Drawing for the job (mm, zero at the part's lowest x, y, z). A direction names the side the tool comes from. Coordinates: 2 decimals unless noted, no trailing zeros. Order: outer loops, then holes, each group sorted by start corner. A loop starts at its lowest first (then second) coordinate and runs counter-clockwise, first axis right, second up.
1) Cut at D-D (x = 9.5). List the corners of the cut face in (y, z).
2) Pin check, flat tips, straight feed: pin 1 Ø2 at (x, z) = (110, 4.5) entering from +Y; pin 2 Ø3 at (x, z) = (20.5, 30.5) entering from -Y; pin 3 Ø1.5 at (x, y) = (98, 18.5) entering from -Z; pin 4 Ø2 at (x, z) = (91, 26) entering from +Y. Stop position of each tip, or through.
3) Wall check: L1, parallel to X at y = 17, z = 19; L2, parallel to Y at x = 111, z = 18.5; L3, parallel to Z at x = 9, y = 24. Give the ranges that are in metal, low to high.
4) Cut at B-B (y = 19.25). List the corners of the cut face in (x, z).
5) Cut at C-C (x = 27.5). List the corners of the cut face in (y, z), and give its area (3 significant figures).
6) Tool access for the marked faces 1 and 2: list every direction of +Z, -Z, +X, -X, +Y, -Y with a clear straight run to the whole face (end or side of a thin tool).
7) Cut at A-A (z = 19.25). List the corners of the cut face in (x, y), and give its area (3 significant figures).
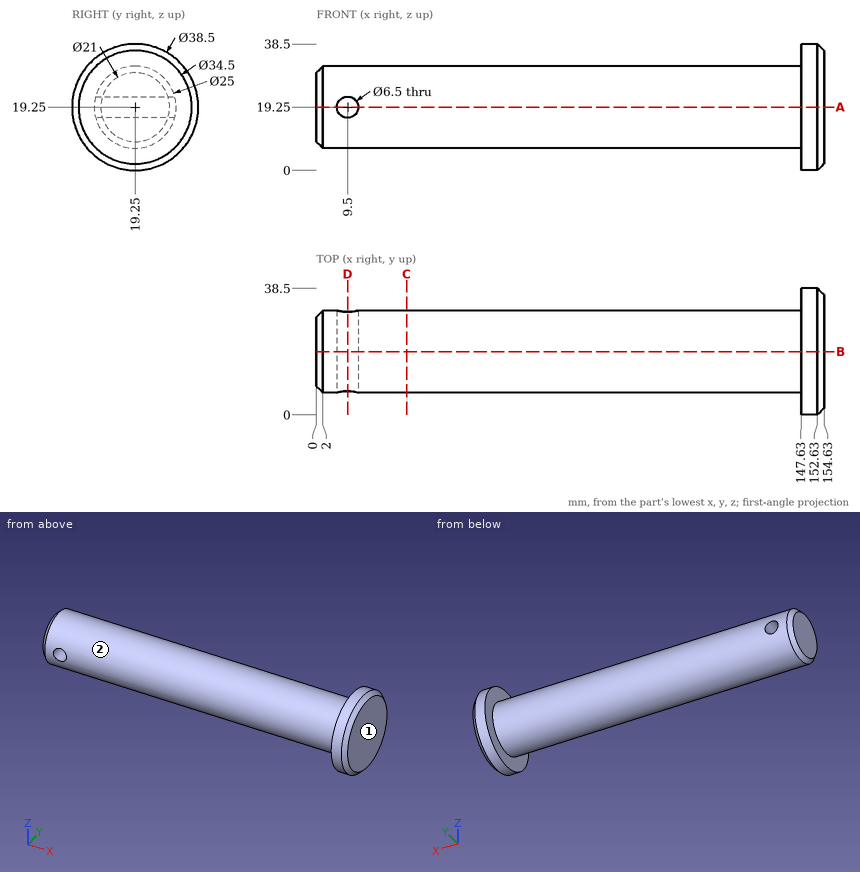
Geometry check:
1. outline: (7.18, 16) arc R12.5 ccw to (31.32, 16) - close; (7.18, 22.5) - (31.32, 22.5) arc R12.5 ccw to start
2. pin 1: passes through
2. pin 2: stops at y = 11.43
2. pin 3: stops at z = 6.75
2. pin 4: stops at y = 30.35
3. L1: x = 0 to 6.26, 12.74 to 154.63
3. L2: y = 6.77 to 31.73
3. L3: z = 7.69 to 16.04, 22.46 to 30.81
4. outline: (0, 8.75) - (2, 6.75) - (147.63, 6.75) - (147.63, 0) - (152.63, 0) - (154.63, 2) - (154.63, 36.5) - (152.63, 38.5) - (147.63, 38.5) - (147.63, 31.75) - (2, 31.75) - (0, 29.75) - close; hole circle Ø6.5 at (9.5, 19.25)
5. outline: circle Ø25 at (19.25, 19.25)
5. area: 491 mm2
6. face 1: +Z, -Z, +X, +Y, -Y
6. face 2: -X
7. outline: (0, 8.75) - (2, 6.75) - (6.25, 6.75) - (6.25, 31.75) - (2, 31.75) - (0, 29.75) - close; (12.75, 6.75) - (147.63, 6.75) - (147.63, 0) - (152.63, 0) - (154.63, 2) - (154.63, 36.5) - (152.63, 38.5) - (147.63, 38.5) - (147.63, 31.75) - (12.75, 31.75) - close
7. area: 3,790 mm2
